Check sheet for the modelled part. Datum: model origin and axes. Units: mm. Round coordinates to 2 decimals unless told otherwise and drop trailing zeros. Loops run counter-clockwise (first coordinate to the right, second up) from the corner with the lowest first, then second, coordinate; pieces in that order, holes last. Notation, with made-up numbers: (81.25, 86) - (114.25, 86) arc R14 cw to (114.25, 91) - close; hole circle Ø11 at (38, 10.25). An arc over 180 degrees is marked (long way). Put each result on its own line as item: value. Start each with the question number.
```python
from build123d import *

# Parameters (mm, degrees)
EXTRUDE_3_DEPTH     = 2000
CUT_EXTRUDE_1_DEPTH = 30


with BuildPart() as part:
    # 草图1 → 凸台-拉伸3 (new body)
    with BuildSketch(Plane(origin=(0, 0, 0), x_dir=(1, 0, 0), z_dir=(0, 1, 0))):
        with BuildLine():
            Line((-1145.538694667, -944.968834947), (-1137.824629383, -938.605408449))
            ThreePointArc((-1137.824629383, -938.605408449), (-1229.702487971, -814.528569836), (-1308.107468768, -681.527585761))
            Line((-1308.107468768, -681.527585761), (-1316.97599398, -686.148111766))
            ThreePointArc((-1316.97599398, -686.148111766), (-1238.039453991, -820.050797428), (-1145.538694667, -944.968834947))
        make_face()
    extrude(amount=EXTRUDE_3_DEPTH)

    # 草图2 → 切除-拉伸1 (cut)
    with BuildSketch(Plane(origin=(0, 0, 0), x_dir=(1, 0, 0), z_dir=(0, 1, 0))):
        with BuildLine():
            Line((-1303.208186932, -699.349284345), (-1304.970469808, -700.294989936))
            ThreePointArc((-1304.970469808, -700.294989936), (-1301.285862357, -707.118168647), (-1297.565579497, -713.921961355))
            Line((-1297.565579497, -713.921961355), (-1295.813296472, -712.957853373))
            ThreePointArc((-1295.813296472, -712.957853373), (-1299.528555318, -706.16324877), (-1303.208186932, -699.349284345))
        make_face()
    extrude(amount=CUT_EXTRUDE_1_DEPTH, mode=Mode.SUBTRACT)


solid = part.part
```
Q1. Material ranges on line 1 (X direction, y = 164.5, z = 825); line 2 (Z direction, x = -1186, y = 1680.5); line 3 (Z direction, x = -1255.5, y = 465), recorded low to high. Write a range as from..to.
Q2. Depth check by flat-ended pin: pin 1 Ø10 at (x, y) = (-1223, 730) entering from +Z; pin 2 Ø1.5 at (x, y) = (-1213, 1478.5) entering from +Z; pin 3 Ø5 at (x, y) = (-1180.5, 940) entering from -Z. Enter the tip coordinate at first touch or a pass-through.
Q3. Cross-section at A-A on y = 639.5. Enter the section's corners in (x, z).
Q4. Cross-section at B-B on z = 863. Enter the section's corners in (x, y), and give its area (3 significant figures).
Answer list:
1. line 1: x = -1234.75..-1222.7
1. line 2: z = 876.94..893.66
1. line 3: z = 774.17..793.06
2. pin 1: stops at z = 849.53
2. pin 2: stops at z = 857.71
2. pin 3: stops at z = 880.99
3. outline: (-1316.98, 686.15) - (-1308.11, 681.53) arc R1475 cw to (-1137.82, 938.61) - (-1145.54, 944.97) arc R1485 ccw to start
4. outline: (-1208.49, 0) - (-1196.18, 0) - (-1196.18, 2000) - (-1208.49, 2000) - close
4. area: 24,600 mm2
